Geometry check sheet. Reference: drawing and pictorial views, mm from the part's lowest x, y, z. A direction names the side the tool comes from. Coordinates: 2 decimals unless noted, no trailing zeros. Loops run counter-clockwise (first coordinate to the right, second up) from the corner with the lowest first, then second, coordinate; pieces in that order, holes last. Notation, with made-up numbers: (-7.5, 20.5) -> (10.5, 20.5) arc R27 ccw to (10.5, 41.5) -> close; hole circle Ø6 at (-1.5, 39). An arc over 180 degrees is marked (long way). Use CSV: the item, a comma, the result in double quotes.
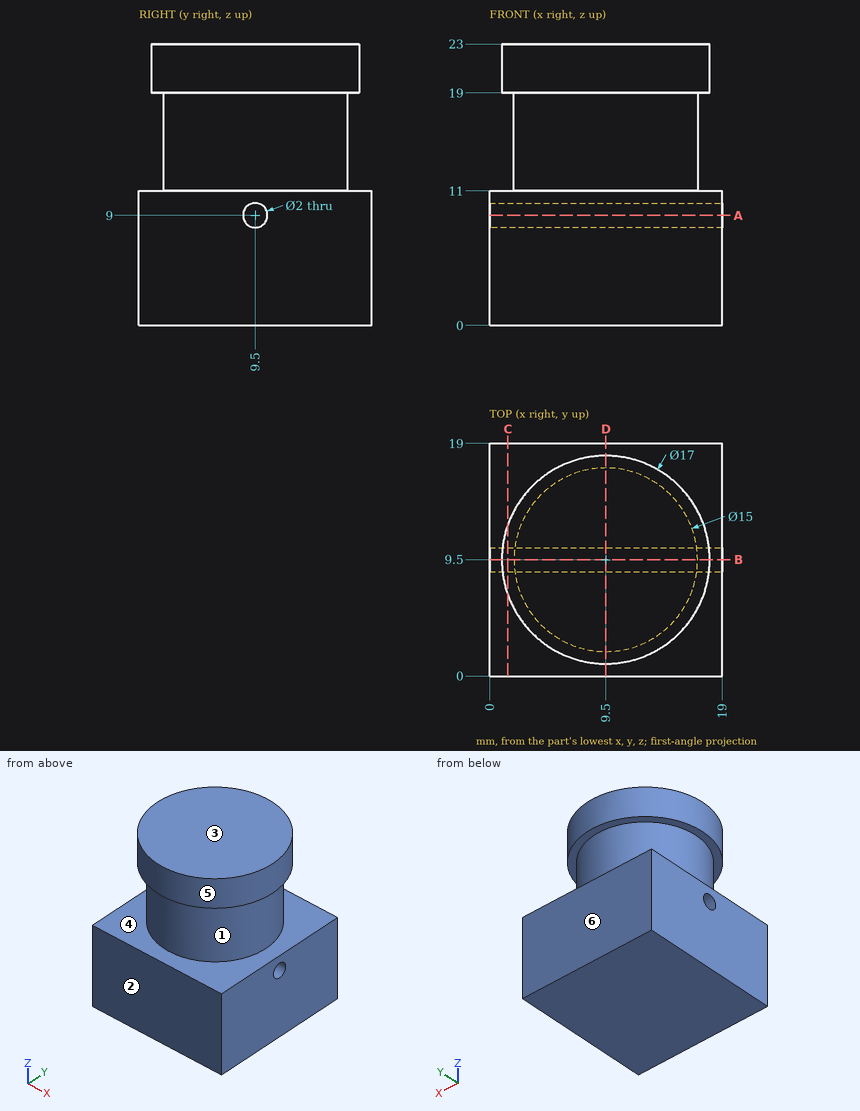
1) Draft check along Z on the marked faces 1, 2, 3 and 4. Enter one of: released by +Z, released by -Z, zero draft, split by the parting line, or undercut.
Answer below:
face 1,"undercut"
face 2,"zero draft"
face 3,"released by +Z"
face 4,"undercut"
2) Cross-section at A-A on z = 9. Record the boundary of the cut face in (x, y), and give its area (3 significant figures).
Answer below:
outline,"(0, 0) -> (19, 0) -> (19, 8.5) -> (0, 8.5) -> close; (0, 10.5) -> (19, 10.5) -> (19, 19) -> (0, 19) -> close"
area,"323 mm²"
3) Access from +Z, -Z, +X, -X, +Y, -Y to the whole of each face (thin tool, end or side, straight path). Record for the marked faces 5 and 6.
Answer below:
face 5,"+Z"
face 6,"+Z, -Z, +X, -X, +Y"
4) Cross-section at D-D on x = 9.5. Record the boundary of the cut face in (y, z).
Answer below:
outline,"(0, 0) -> (19, 0) -> (19, 11) -> (17, 11) -> (17, 19) -> (18, 19) -> (18, 23) -> (1, 23) -> (1, 19) -> (2, 19) -> (2, 11) -> (0, 11) -> close; hole circle Ø2 at (9.5, 9)"
5) Thickness scan on line 1 along Y through (x, z) = (11.25, 9); line 2 along Z through (x, y) = (16.5, 6.5); line 3 along Z through (x, y) = (7.75, 18). Record the ranges inside material, lowest first. Write a range as from..to.
Answer below:
line 1,"y = 0..8.5, 10.5..19"
line 2,"z = 0..11, 19..23"
line 3,"z = 0..11"
6) Go/stop test with flat-tipped pins: pin 1 Ø1 at (y, z) = (16.5, 14) entering from +X; pin 2 Ø5 at (x, z) = (13.5, 15) entering from -Y. Record where each tip stops, or that it passes through.
Answer below:
pin 1,"stops at x = 13.24"
pin 2,"stops at y = 2.15"
7) Cross-section at C-C on x = 1.5. Record the boundary of the cut face in (y, z).
Answer below:
outline,"(0, 0) -> (19, 0) -> (19, 11) -> (0, 11) -> close; (6.63, 19) -> (12.37, 19) -> (12.37, 23) -> (6.63, 23) -> close; hole circle Ø2 at (9.5, 9)"
8) Cross-section at B-B on y = 9.5. Record the boundary of the cut face in (x, z).
Answer below:
outline,"(0, 0) -> (19, 0) -> (19, 8) -> (0, 8) -> close; (0, 10) -> (19, 10) -> (19, 11) -> (17, 11) -> (17, 19) -> (18, 19) -> (18, 23) -> (1, 23) -> (1, 19) -> (2, 19) -> (2, 11) -> (0, 11) -> close"
